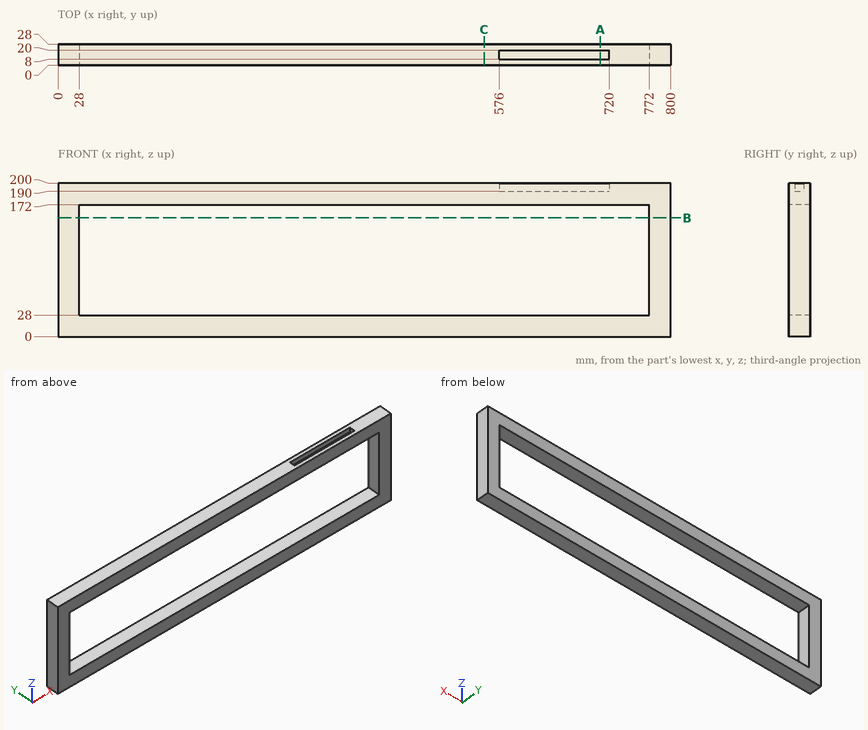
Drawing for the job (mm, zero at the part's lowest x, y, z). Round coordinates to 2 decimals unless told otherwise and drop trailing zeros. Write each loop counter-clockwise with the first axis right and the second up, starting at its lowest first coordinate (ties: lowest second). Pieces come first, ordered by that corner, then holes. Notation, with made-up numbers: M 46.5,52.25 L 64.5,52.25 A27 ccw 64.5,79.25 Z; hole C -12.5,22 d6. An arc over 180 degrees is marked long. Answer as a JSON object with one key per item and string values. Group by question number.
(1) Drill centre lines: L1, parallel to X at y = 12.75, z = 40; L2, parallel to Z at x = 657, y = 16.25; L3, parallel to Z at x = 420.5, y = 13.75. Where is each one in solid material? Low to high.
(2) Cut at A-A (x = 708.5). Give the cut face in (y, z).
(3) Cut at B-B (z = 155). Give the cut face in (x, y).
(4) Cut at C-C (x = 556.5). Give the cut face in (y, z), and give its area (3 significant figures).
(5) Flat gauge pins, fed straight in: pin 1 (8.5 mm diameter, centred on y = 20.5, z = 88, fed in from -X); pin 2 (3.5 mm diameter, centred on x = 627.5, y = 13, fed in from +Z). Where does each tip first touch, or does it go through?
Responses:
{
 "1": {"L1": "x = 0 to 28, 772 to 800", "L2": "z = 0 to 28, 172 to 190", "L3": "z = 0 to 28, 172 to 200"},
 "2": {"outline": "M 0,0 L 28,0 L 28,28 L 0,28 Z; M 0,172 L 28,172 L 28,200 L 20,200 L 20,190 L 8,190 L 8,200 L 0,200 Z"},
 "3": {"outline": "M 0,0 L 28,0 L 28,28 L 0,28 Z; M 772,0 L 800,0 L 800,28 L 772,28 Z"},
 "4": {"outline": "M 0,0 L 28,0 L 28,28 L 0,28 Z; M 0,172 L 28,172 L 28,200 L 0,200 Z", "area": "1,570 mm2"},
 "5": {"pin 1": "stops at x = 0", "pin 2": "stops at z = 190"}
}
